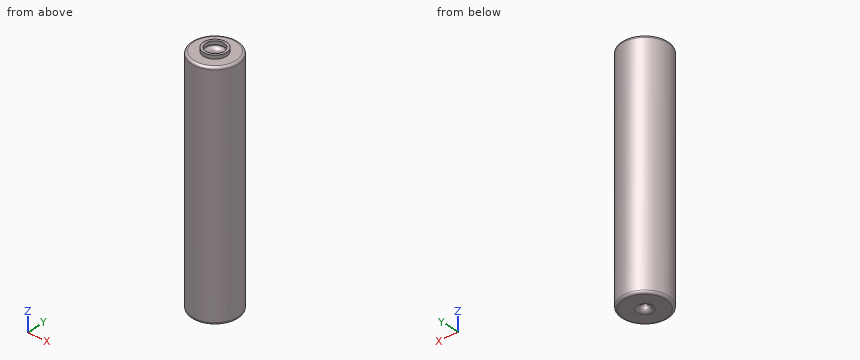
```python
from build123d import *


with BuildPart() as part:
    # Sketch → Revolution (revolve)
    with BuildSketch(Plane.YZ):
        with BuildLine():
            Line((-1.5, 5), (-1.5, 2))
            ThreePointArc((-3.5, 0), (-2.085786, 0.585786), (-1.5, 2))
            Line((-3.5, 0), (-9, 0))
            ThreePointArc((-10, 1), (-9.707107, 0.292893), (-9, 0))
            Line((-10, 1), (-10, 99))
            ThreePointArc((-9, 100), (-9.707107, 99.707107), (-10, 99))
            Line((-9, 100), (-4.95, 100))
            Line((-4.95, 100), (-4.95, 101.5))
            Line((-4.95, 101.5), (-3.95, 101.5))
            Line((-3.95, 101.5), (-3.95, 100))
            Line((-3.95, 100), (-3.499999, 100))
            ThreePointArc((-1.5, 98), (-2.085786, 99.414213), (-3.499999, 100))
            Line((-1.5, 98), (-1.5, 95))
            Line((-1.5, 95), (-8.25, 80.524578))
            Line((-8.25, 80.524578), (-8.25, 19.475422))
            Line((-1.5, 5), (-8.25, 19.475422))
        make_face()
    revolve(axis=Axis((0, 0, 0), (0, 0, 1)))


solid = part.part
```
Input: part model. Units: mm. Frame: model coordinates. Give positions to 0.01 mm unless a question says otherwise; leave off trailing zeros. Loops run counter-clockwise (first coordinate to the right, second up) from the corner with the lowest first, then second, coordinate; pieces in that order, holes last. Notation, with made-up numbers: (33, -37.75) -> (89, -37.75) arc R23 cw to (89, -26.75) -> close; hole circle Ø5 at (-13, -9.75). An arc over 180 degrees is marked (long way). Use a Markdown table: item, result.
Q1. First-contact query: P1, Ø2, axis at x = 5, z = 11.5, coming from the +Y side; P2, Ø8, axis at y = 7.5, z = 29.5, coming from the +X side; P3, Ø5, axis at x = -3.5, z = 71.5, coming from the +Y side; P4, Ø8, axis at x = 1, z = 59, coming from the -Y side. Flat tips, straight axial feed; report the tip coordinate or a pass-through.
Entries:
| item | result |
|---|---|
| P1 | stops at y = 9.17 |
| P2 | stops at x = 9.37 |
| P3 | stops at y = 9.95 |
| P4 | stops at y = -10 |
Q2. Ray query, probe 1 along X at (y, z) = (0, 3.55); probe 2 along X at (y, z) = (0, 62); probe 3 along Z at (x, y) = (-6, 4.5). Return the intervals inside material, ascending. Write a range as from..to.
Entries:
| item | result |
|---|---|
| probe 1 | x = -10..-1.5, 1.5..10 |
| probe 2 | x = -10..-8.25, 8.25..10 |
| probe 3 | z = 0..17.87, 82.13..100 |
Q3. Section query C-C, the plane z = 35.5. Return the cut outline in (x, y).
Entries:
| item | result |
|---|---|
| outline | circle Ø20 at (0, 0); hole circle Ø16.5 at (0, 0) |
Q4. Section query D-D, the plane z = 88. Return the cut outline in (x, y).
Entries:
| item | result |
|---|---|
| outline | circle Ø20 at (0, 0); hole circle Ø9.53 at (0, 0) |
